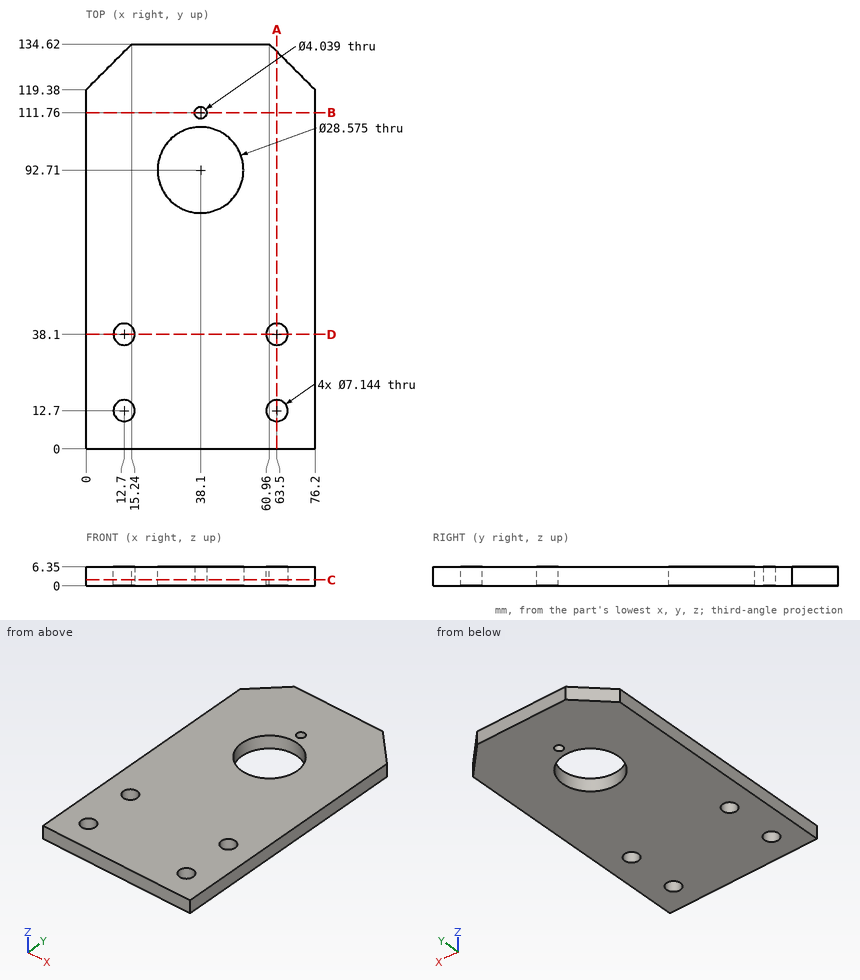
Part print with two shaded views. Sizes in mm from the minimum x, y, z corner. Round coordinates to 2 decimals unless told otherwise and drop trailing zeros. Write each loop counter-clockwise with the first axis right and the second up, starting at its lowest first coordinate (ties: lowest second). Pieces come first, ordered by that corner, then holes. Notation, with made-up numbers: (-1, -16) - (20, -16) arc R26 cw to (20, 21) - close; hole circle Ø9 at (-22.75, -24.5). An arc over 180 degrees is marked (long way). Answer as CSV lines item,"result".
Q1. Cut at B-B (y = 111.76). Write the cut outline in (x, z), and give its area (3 significant figures).
Report:
outline,"(0, 0) - (36.08, 0) - (36.08, 6.35) - (0, 6.35) - close; (40.12, 0) - (76.2, 0) - (76.2, 6.35) - (40.12, 6.35) - close"
area,"458 mm^2"
Q2. Drop a flat-ended pin along its axis: pin 1 (1.5 mm diameter, centred on y = 120.5, z = 2, fed in from -X). Give the stop position or say it passes through.
Report:
pin 1,"stops at x = 0.37"
Q3. Cut at D-D (y = 38.1). Write the cut outline in (x, z).
Report:
outline,"(0, 0) - (9.13, 0) - (9.13, 6.35) - (0, 6.35) - close; (16.27, 0) - (59.93, 0) - (59.93, 6.35) - (16.27, 6.35) - close; (67.07, 0) - (76.2, 0) - (76.2, 6.35) - (67.07, 6.35) - close"
Q4. Cut at A-A (x = 63.5). Write the cut outline in (y, z).
Report:
outline,"(0, 0) - (9.13, 0) - (9.13, 6.35) - (0, 6.35) - close; (16.27, 0) - (34.53, 0) - (34.53, 6.35) - (16.27, 6.35) - close; (41.67, 0) - (132.08, 0) - (132.08, 6.35) - (41.67, 6.35) - close"
Q5. Cut at C-C (z = 2). Write the cut outline in (x, y) (1 decimal), and give its area (3 significant figures).
Report:
outline,"(0, 0) - (76.2, 0) - (76.2, 119.4) - (61, 134.6) - (15.2, 134.6) - (0, 119.4) - close; hole circle Ø7.1 at (12.7, 12.7); hole circle Ø7.1 at (12.7, 38.1); hole circle Ø28.6 at (38.1, 92.7); hole circle Ø4 at (38.1, 111.8); hole circle Ø7.1 at (63.5, 12.7); hole circle Ø7.1 at (63.5, 38.1)"
area,"9,210 mm^2"
Q6. Drill centre lines: probe 1 along Y at (x, z) = (38.1, 4.75); probe 2 along Y at (x, z) = (63.5, 2.25); probe 3 along Y at (x, z) = (34, 4). Where is each one in solid material? Low to high. Write a range as [from, to].
Report:
probe 1,"y = [0, 78.42], [107, 109.74], [113.78, 134.62]"
probe 2,"y = [0, 9.13], [16.27, 34.53], [41.67, 132.08]"
probe 3,"y = [0, 79.02], [106.4, 134.62]"
